The listing builds one solid part. Answer for the finished solid, in the listing's coordinates (mm). Face numbers are marked on the shaded views. A direction names the side the tool comes from. Coordinates: 2 decimals unless noted, no trailing zeros. Loops run counter-clockwise (first coordinate to the right, second up) from the corner with the lowest first, then second, coordinate; pieces in that order, holes last. Notation, with made-up numbers: M 28.25,-34 L 39.25,-34 A17 cw 39.25,-12 Z; hole C 33,41 d3. An arc over 180 degrees is marked long. Answer in a Markdown table with one row per item. Add a question column.
from build123d import *

# Parameters (mm, degrees)
F1_DEPTH = 10


with BuildPart() as f1:
    # F0 (on Front) → F1 (new body)
    with BuildSketch(Plane.XZ):
        with BuildLine():
            ThreePointArc((-26.480538, 0.041752), (-26.80275, -6.984853), (-24.610945, -13.66864))
            Line((-24.610945, -13.66864), (9.389055, -13.66864))
            ThreePointArc((9.389055, -13.66864), (11.76884, -7.015264), (11.409232, 0.041752))
            ThreePointArc((11.409232, 0.041752), (9.53605, 1.729011), (7.207622, 0.762533))
            Line((7.207622, 0.762533), (5.26171, -2.592488))
            Line((5.26171, -2.592488), (6.516005, -3.31998))
            Line((6.516005, -3.31998), (8.512528, 0.122302))
            ThreePointArc((8.512528, 0.122302), (8.872618, 0.286233), (9.145764, 0))
            ThreePointArc((9.145764, 0), (9.12048, -3.50336), (7.994913, -6.821081))
            ThreePointArc((7.994913, -6.821081), (3.623874, -11.160444), (-0.715488, -6.789405))
            ThreePointArc((-0.715488, -6.789405), (-2.12155, -3.515707), (-1.92509, 0.041752))
            ThreePointArc((-1.92509, 0.041752), (-1.611125, 0.372473), (-1.205894, 0.163336))
            Line((-1.205894, 0.163336), (0.535578, -3.437674))
            Line((0.535578, -3.437674), (1.840945, -2.80639))
            Line((1.840945, -2.80639), (0.099355, 0.794863))
            ThreePointArc((0.099355, 0.794863), (-1.83955, 2.01093), (-3.778454, 0.794863))
            Line((-3.778454, 0.794863), (-5.72786, -2.673798))
            ThreePointArc((-5.72786, -2.673798), (-7.366983, -3.479416), (-9.006107, -2.673798))
            Line((-9.006107, -2.673798), (-11.616714, 1.475432))
            ThreePointArc((-11.616714, 1.475432), (-13.425926, 2.377495), (-15.235137, 1.475432))
            Line((-15.235137, 1.475432), (-17.64233, -1.719161))
            Line((-17.64233, -1.719161), (-16.48429, -2.591769))
            Line((-16.48429, -2.591769), (-14.077097, 0.602824))
            ThreePointArc((-14.077097, 0.602824), (-13.524899, 0.812886), (-13.096491, 0.406049))
            ThreePointArc((-13.096491, 0.406049), (-12.908327, -3.030287), (-14.181236, -6.22771))
            Line((-14.181236, -6.22771), (-14.176145, -6.414763))
            ThreePointArc((-14.176145, -6.414763), (-18.316139, -10.926878), (-22.956589, -6.931259))
            ThreePointArc((-22.956589, -6.931259), (-24.297873, -3.334327), (-24.321447, 0.504476))
            ThreePointArc((-24.321447, 0.504476), (-24.044014, 0.761092), (-23.700835, 0.602824))
            Line((-23.700835, 0.602824), (-21.668322, -2.716693))
            Line((-21.668322, -2.716693), (-20.431714, -1.959527))
            Line((-20.431714, -1.959527), (-22.51379, 1.440936))
            ThreePointArc((-22.51379, 1.440936), (-24.932699, 1.976107), (-26.480538, 0.041752))
        make_face()
    extrude(amount=F1_DEPTH)


solid = f1.part
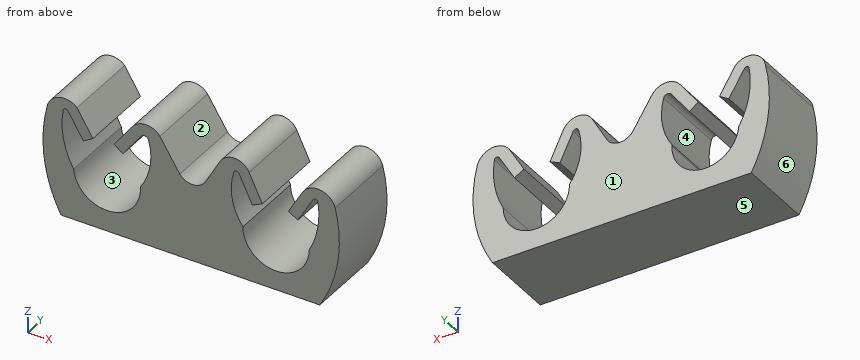
(1) Straight lines are drawn through the part: line 1 (X direction, y = -4.75, z = -4.75); line 2 (X direction, y = -7.75, z = -7); line 3 (Z direction, x = -14, y = -9). For each, find the intervals that lie inside material, in ascending order.
(2) For the marked faces 1, 2 and 3, determine the directions among +Z, -Z, +X, -X, +Y, -Y from which every point of the face is accessible in a straight line to the end or side of a thin tool.
(3) Each of these flat-tipped pins is pushed along its axis until it touches: pin 1 (1 mm diameter, centred on y = -8.5, z = -3.5, fed in from +X); pin 2 (2 mm diameter, centred on x = 4, z = -10, fed in from +Y); pin 3 (4 mm diameter, centred on x = -15, y = -2.5, fed in from +Z). Where does it stop, or does it pass through?
(4) A cutting plane is placed at D-D (z = -9.75). Give the vertices of the cut face in (x, y), plus the area to 3 significant figures.
(5) A cutting plane is placed at A-A (z = -5.25). Give the vertices of the cut face in (x, y).
(6) The mould has two halves that part along X. Classify the marked faces 4, 5 and 6: released by +X, released by -X, zero draft, split by the parting line, or undercut.
(7) A cutting plane is placed at C-C (z = -1.25). State how many separate pieces and enclosed holes the cut face has, plus the area to 3 significant figures.
Solved:
| question | item | result |
|---|---|---|
| 1 | line 1 | x = -26.98 to -23.94, -13.39 to -1.8, 8.83 to 11.96 |
| 1 | line 2 | x = -26.8 to -22.95, -14.2 to -0.71, 7.99 to 11.77 |
| 1 | line 3 | z = -13.67 to -5.95, 0.69 to 2.3 |
| 2 | face 1 | +Z, -Z, +X, -X, +Y |
| 2 | face 2 | +Z, +Y, -Y |
| 2 | face 3 | +Y, -Y |
| 3 | pin 1 | stops at x = 11.96 |
| 3 | pin 2 | passes through |
| 3 | pin 3 | stops at z = 2.38 |
| 4 | outline | M -26.22,-10 L -21.58,-10 L -21.58,0 L -26.22,0 Z; M -15.57,-10 L 0.43,-10 L 0.43,0 L -15.57,0 Z; M 6.85,-10 L 11.15,-10 L 11.15,0 L 6.85,0 Z |
| 4 | area | 249 mm² |
| 5 | outline | M -26.96,-10 L -23.76,-10 L -23.76,0 L -26.96,0 Z; M -13.61,-10 L -1.6,-10 L -1.6,0 L -13.61,0 Z; M 8.68,-10 L 11.94,-10 L 11.94,0 L 8.68,0 Z |
| 6 | face 4 | undercut |
| 6 | face 5 | zero draft |
| 6 | face 6 | released by -X |
| 7 | separate pieces | 8 |
| 7 | enclosed holes | 0 |
| 7 | area | 171 mm² |
